Autodesk Inventor part; units mm, degrees
ref_plane "YZ Plane" through (0, 0, 0) normal (1, 0, 0) x (0, 1, 0)
ref_plane "XZ Plane" through (0, 0, 0) normal (0, 1, 0) x (-1, 0, 0)
ref_plane "XY Plane" through (0, 0, 0) normal (0, 0, 1) x (1, 0, 0)
sketch "Sketch1" plane through (0, 0, 0) normal (0, 0, 1) x (1, 0, 0)
  circle A0 centre (0, 0) radius 1.5
  circle A1 centre (0, 0) radius 4
  circle A2 centre (0, 0) radius 7 construction
  line L0 (0, 0) -> (0, 7) construction
  circle A3 centre (-1, 13.3125) radius 6.35
  line L1 (0, 0) -> (0, 7) construction
  line L2 (4, 0) -> (4, 7)
  line L3 (-4, 7) -> (-4, 0)
  arc A4 (-4, 0) -> (4, 0) centre (0, 0) ccw
  arc A5 (4, 7) -> (-4, 7) centre (0, 7) ccw
  point P0 (0, 3.5)
  point P1 (-3.9251, 7.7702)
  point P2 (4, 0)
  point P3 (3.5364, 8.8691)
  point P4 (-4, 0)
  point P5 (-3.941, 7.6846)
  dimension "d2" = 14
  dimension "d0" = 3
  dimension "d1" = 8
  dimension "d3" = 12.7
  dimension "d4" = 4
  dimension "d9" = 1
extrude "Extrusion1" add sketch "Sketch1" along normal blind 4.7625 contours A1 | A1 L3 A5 A3 L2
fillet "Fillet1" radius 1.5 2 edges at (3.5364, 8.8691, 2.3813) (-3.941, 7.6846, 2.3813)
sketch "Sketch2" plane through (0, 0, 0) normal (0, 0, -1) x (-1, 0, 0)
  arc A0 (4, 5.6071) -> (2.2134, 7.0795) centre (2.5, 5.6071) ccw
  arc A1 (-1.8312, 7.6286) -> (2.2134, 7.0795) centre (1, 13.3125) ccw
  arc A2 (-1.8312, 7.6286) -> (-4, 6.2859) centre (-2.5, 6.2859) ccw
  line L0 (-4, 0) -> (-4, 6.2859)
  arc A3 (-4, 0) -> (4, 0) centre (0, 0) ccw
  line L1 (4, 5.6071) -> (4, 0)
  circle A4 centre (0, 0) radius 1.5
  circle A5 centre (0, 0) radius 8.2648 construction
equation "\"d4\" = 0.5 * d1"
properties part number "Cam - Lever" material "Nylon 6/6"
Design review of the part built by this model. Coordinates are the model's own, in mm. Round coordinates to 2 decimals unless told otherwise and drop trailing zeros. Order: outer loops, then holes, each group sorted by start corner. A loop starts at its lowest first (then second) coordinate and runs counter-clockwise, first axis right, second up.
1) Consider section B-B (x = -0.25). State the section outline as (y, z) points.
The answers:
outline: (-3.99, 0) - (-1.48, 0) - (-1.48, 4.76) - (-3.99, 4.76) - close; (1.48, 0) - (7.01, 0) - (7.01, 4.76) - (1.48, 4.76) - close
2) For L1, parallel to Y at x = -0.75, z = 2.65; L2, parallel to Y at x = -1, z = 3.7; L3, parallel to X at y = 1.25, z = 0.8, list the stretches that pass through material, from the lowest coordinate up.
The answers:
L1: y = -3.93 to -1.3, 1.3 to 6.97
L2: y = -3.87 to -1.12, 1.12 to 6.96
L3: x = -4 to -0.83, 0.83 to 4
3) Consider section D-D (x = -1.75). State the section outline as (y, z) points.
The answers:
outline: (-3.6, 0) - (7.01, 0) - (7.01, 4.76) - (-3.6, 4.76) - close
4) Draft analysis for pull direction X (two halves, no side actions). For faces 1 (the cylindrical face through (0, -4, 2)), 2 (the cylindrical face through (-1.5, -0.07, 2.35)), 3 (the flat face through (0, 2, 4.762)), state which applies: released by +X, released by -X, zero draft, split by the parting line, or undercut.
The answers:
face 1: split by the parting line
face 2: undercut
face 3: zero draft
5) Consider section C-C (y = -2.75). State the section outline as (x, z) points, plus the area to 3 significant figures.
The answers:
outline: (-2.9, 0) - (2.9, 0) - (2.9, 4.76) - (-2.9, 4.76) - close
area: 27.7 mm2
6) Consider section A-A (x = 0.75). State the section outline as (y, z) points.
The answers:
outline: (-3.93, 0) - (-1.3, 0) - (-1.3, 4.76) - (-3.93, 4.76) - close; (1.3, 0) - (7.21, 0) - (7.21, 4.76) - (1.3, 4.76) - close
